Build history of the part. All positions in model axes, mm. Face numbers are marked on the shaded views. A direction names the side the tool comes from. Round coordinates to 2 decimals unless told otherwise and drop trailing zeros. Write each loop counter-clockwise with the first axis right and the second up, starting at its lowest first coordinate (ties: lowest second). Pieces come first, ordered by that corner, then holes.
1) Saw through at D-D (y = -4.75). Write the cut outline in (x, z).
2) Pull direction Y, two halves, no side cores. Call the marked faces 6, 7, 8 and 9: +Y half, -Y half, draft (parallel to the pull), parting line (faces both ways), or undercut.
3) Flat gauge pins, fed straight in: pin 1 (1.8 mm diameter, centred on x = -1, z = 2, fed in from +Y); pin 2 (2 mm diameter, centred on y = -8, z = 4, fed in from -X); pin 3 (3 mm diameter, centred on y = 3, z = 2.5, fed in from -X). Where does each tip first touch, or does it go through?
4) Saw through at A-A (x = -7.25). Write the cut outline in (y, z), plus the area to 3 significant figures.
5) Which spindle directions (+Z, -Z, +X, -X, +Y, -Y) get a long thin tool onto all of the face, cutting with end or side? Do the marked faces 1, 2, 3, 4 and 5. Say none if no direction does.
6) Saw through at C-C (y = -9). Write the cut outline in (x, z).
7) Saw through at B-B (y = 7.75). Write the cut outline in (x, z), plus the area to 3 significant figures.
8) Wall check: probe 1 along Y at (x, z) = (-7.25, 3.3); probe 2 along Y at (x, z) = (8.5, 1.45); probe 3 along X at (y, z) = (8, 0.6). Give the ranges that are in metal, low to high.
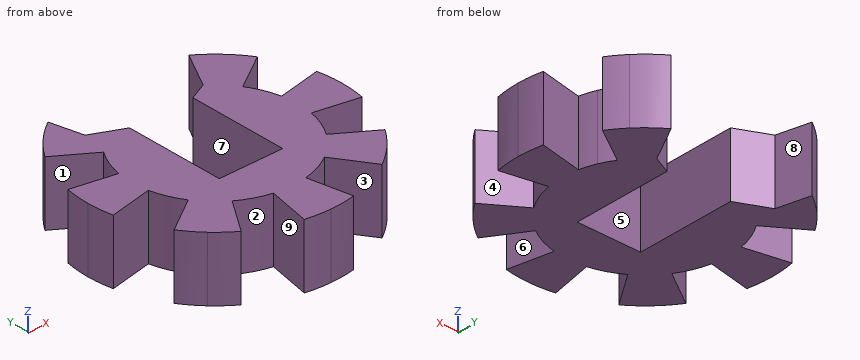
from build123d import *

# Parameters (mm, degrees)
RESSALTO_EXTRUS_O1_DEPTH = 6


with BuildPart() as part:
    # Esboço1 → Ressalto-extrusão1 (new body)
    with BuildSketch(Plane.XY):
        with BuildLine():
            Line((-3, -3.719131056), (3, -3.719131056))
            Line((3, -3.719131056), (3, 5.552723944))
            Line((3, 5.552723944), (4.686976687, 6.338438926))
            Line((4.686976687, 6.338438926), (6.666842796, 9.977635348))
            ThreePointArc((6.666842796, 9.977635348), (7.823592894, 9.098977648), (8.865699639, 8.08698769))
            ThreePointArc((8.865699639, 8.08698769), (9.481878586, 7.354860874), (10.037762914, 6.575965))
            Line((10.037762914, 6.575965), (6.572308916, 4.305667884))
            ThreePointArc((6.572308916, 4.305667884), (6.946088732, 3.672311498), (7.259013875, 3.006781996))
            ThreePointArc((7.259013875, 3.006781996), (7.518775912, 2.280795738), (7.706128027, 1.532844169))
            Line((7.706128027, 1.532844169), (11.769423365, 2.341083864))
            ThreePointArc((11.769423365, 2.341083864), (11.94221672, 1.176205684), (12, 0))
            ThreePointArc((12, 0), (11.94221672, -1.176205684), (11.769423365, -2.341083864))
            Line((11.769423365, -2.341083864), (7.706128027, -1.532844169))
            ThreePointArc((7.706128027, -1.532844169), (7.259013875, -3.006781996), (6.532939891, -4.365170878))
            Line((6.532939891, -4.365170878), (9.977635348, -6.666842796))
            ThreePointArc((9.977635348, -6.666842796), (9.27612544, -7.61271941), (8.485281374, -8.485281374))
            ThreePointArc((8.485281374, -8.485281374), (7.61271941, -9.27612544), (6.666842796, -9.977635348))
            Line((6.666842796, -9.977635348), (4.365170878, -6.532939891))
            ThreePointArc((4.365170878, -6.532939891), (3.006781996, -7.259013875), (1.532844169, -7.706128027))
            Line((1.532844169, -7.706128027), (2.341083864, -11.769423365))
            ThreePointArc((2.341083864, -11.769423365), (1.176205684, -11.94221672), (0, -12))
            ThreePointArc((0, -12), (-1.176205684, -11.94221672), (-2.341083864, -11.769423365))
            Line((-2.341083864, -11.769423365), (-1.532844169, -7.706128027))
            ThreePointArc((-1.532844169, -7.706128027), (-3.006781996, -7.259013875), (-4.365170878, -6.532939891))
            Line((-4.365170878, -6.532939891), (-6.666842796, -9.977635348))
            ThreePointArc((-6.666842796, -9.977635348), (-7.61271941, -9.27612544), (-8.485281374, -8.485281374))
            ThreePointArc((-8.485281374, -8.485281374), (-9.27612544, -7.61271941), (-9.977635348, -6.666842796))
            Line((-9.977635348, -6.666842796), (-6.532939891, -4.365170878))
            ThreePointArc((-6.532939891, -4.365170878), (-7.259013875, -3.006781996), (-7.706128027, -1.532844169))
            Line((-7.706128027, -1.532844169), (-11.769423365, -2.341083864))
            ThreePointArc((-11.769423365, -2.341083864), (-11.94221672, -1.176205684), (-12, 0))
            ThreePointArc((-12, 0), (-11.94221672, 1.176205684), (-11.769423365, 2.341083864))
            Line((-11.769423365, 2.341083864), (-7.706128027, 1.532844169))
            ThreePointArc((-7.706128027, 1.532844169), (-7.259013875, 3.006781996), (-6.532939891, 4.365170878))
            Line((-6.532939891, 4.365170878), (-9.977635348, 6.666842796))
            ThreePointArc((-9.977635348, 6.666842796), (-9.27612544, 7.61271941), (-8.485281374, 8.485281374))
            ThreePointArc((-8.485281374, 8.485281374), (-7.61271941, 9.27612544), (-6.666842796, 9.977635348))
            Line((-6.666842796, 9.977635348), (-5.941249609, 6.922620695))
            Line((-5.941249609, 6.922620695), (-3, 5.552723944))
            Line((-3, 5.552723944), (-3, -3.719131056))
        make_face()
    extrude(amount=RESSALTO_EXTRUS_O1_DEPTH)


solid = part.part
Evaluation:
1. outline: (-7.11, 0) - (7.11, 0) - (7.11, 6) - (-7.11, 6) - close
2. face 6: undercut
2. face 7: draft
2. face 8: +Y half
2. face 9: undercut
3. pin 1: stops at y = -3.72
3. pin 2: stops at x = -9.75
3. pin 3: stops at x = -11.91
4. outline: (-9.56, 0) - (-4.84, 0) - (-4.84, 6) - (-9.56, 6) - close; (-3.03, 0) - (3.03, 0) - (3.03, 6) - (-3.03, 6) - close; (4.84, 0) - (9.56, 0) - (9.56, 6) - (4.84, 6) - close
4. area: 93.0 mm2
5. face 1: +Z, -Z, -X
5. face 2: +Z, -Z
5. face 3: +Z, -Z, -Y
5. face 4: +Z, -Z, +X
5. face 5: +Z, -Z, +Y
6. outline: (-7.94, 0) - (-6.01, 0) - (-6.01, 6) - (-7.94, 6) - close; (-1.79, 0) - (1.79, 0) - (1.79, 6) - (-1.79, 6) - close; (6.01, 0) - (7.94, 0) - (7.94, 6) - (6.01, 6) - close
7. outline: (-9.16, 0) - (-6.14, 0) - (-6.14, 6) - (-9.16, 6) - close; (5.45, 0) - (9.16, 0) - (9.16, 6) - (5.45, 6) - close
7. area: 40.4 mm2
8. probe 1: y = -9.56 to -4.84, -3.03 to 3.03, 4.84 to 9.56
8. probe 2: y = -8.47 to -5.68, -1.69 to 1.69, 5.57 to 8.47
8. probe 3: x = -8.94 to -6.2, 5.59 to 8.94
